Input: part model. Units: mm. Frame: model coordinates. Face numbers are marked on the shaded views. A direction names the side the tool comes from. Give positions to 0.01 mm unless a question says otherwise; leave off trailing zeros. Loops run counter-clockwise (first coordinate to the right, second up) from the corner with the lowest first, then second, coordinate; pieces in that order, holes last. Notation, with made-up numbers: M 9,42 L 51,42 A14 ccw 51,56 Z; hole C -39,6.25 d9. An arc over 180 degrees is marked long. One line per item, written item: value. Start each with the question number.
(1) Ray query, line 1 along X through (y, z) = (25, 0); line 2 along X through (y, z) = (33, -35); line 3 along Y through (x, z) = (0, 47.35). Return the intervals inside material, ascending. Write a range as from..to.
(2) Section A-A on y = 39.5. Output: boundary loops of the cut face in (x, z), plus the area to 3 significant figures.
(3) Section D-D on x = -17. Output: boundary loops of the cut face in (y, z), plus the area to 3 significant figures.
(4) Access query for the marked faces 1, 2 and 3. Directions: +Z, -Z, +X, -X, +Y, -Y. A direction counts if a zero-diameter tool reaches every point of the face in a straight line with its end or side. Return the directions, or none.
(5) Pull-direction query (X, two-part tool) for the marked faces 4, 5, 6 and 7; classes: released by +X, released by -X, zero draft, split by the parting line, or undercut.
(6) Section B-B on z = 0. Output: boundary loops of the cut face in (x, y).
(7) Pin query (flat end, axial travel): P1, Ø10.5, axis at x = -8.5, z = 21.5, coming from the +Y side; P2, Ø1, axis at y = 48.5, z = 14, coming from the +X side; P3, Ø22, axis at x = 3, y = 19.5, coming from the +Z side. Return the tip coordinate at first contact, or that it passes through.
(8) Section C-C on z = -41. Output: boundary loops of the cut face in (x, y), plus the area to 3 significant figures.
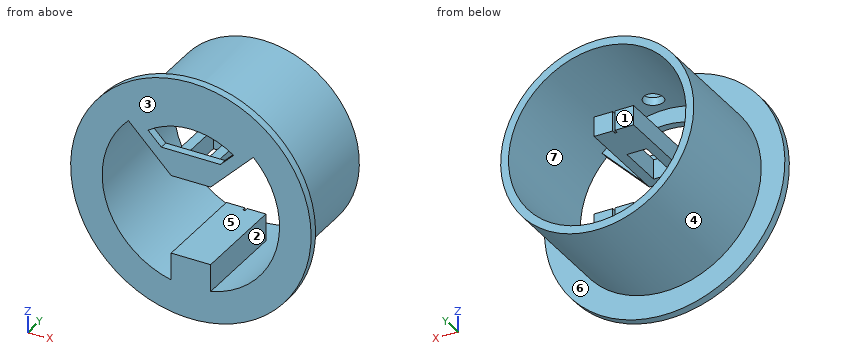
```python
from build123d import *

# Parameters (mm, degrees)
SKETCH1_R               = 61
SKETCH1_R_2             = 49
BOSS_EXTRUDE1_DEPTH     = 4
BOSS_EXTRUDE2_DEPTH     = 4
SKETCH1_5_R             = 49
SKETCH1_5_R_2           = 45
BOSS_EXTRUDE3_DEPTH     = 64.4
SKETCH1_8_W             = 20
SKETCH1_8_H             = 10
BOSS_EXTRUDE4_DEPTH     = 49.5
CUT_EXTRUDE1_REACH      = 115.669
SKETCH2_W               = 10
SKETCH2_H               = 24
CUT_EXTRUDE2_REACH      = 115.669
CUT_EXTRUDE2_END_RADIUS = 49
SKETCH3_R               = 5
CUT_EXTRUDE4_START      = -2
CUT_EXTRUDE4_DEPTH      = 2
SKETCH5_W               = 1.2
SKETCH5_H               = 10
CUT_EXTRUDE5_DEPTH      = 2


with BuildPart() as part:
    # Sketch1 → Boss-Extrude1 (new body)
    with BuildSketch(Plane(origin=(0, 0, 0), x_dir=(1, 0, 0), z_dir=(0, 1, 0))):
        with Locations(Location((0, 0, 0), (0, 0, 270))):
            Circle(SKETCH1_R)
        with Locations(Location((0, 0, 0), (0, 0, 270))):
            Circle(SKETCH1_R_2, mode=Mode.SUBTRACT)
    extrude(amount=BOSS_EXTRUDE1_DEPTH)



with BuildPart() as body_2:
    # Sketch1<4> → Boss-Extrude2 (new body)
    with BuildSketch(Plane(origin=(0, 0, 0), x_dir=(1, 0, 0), z_dir=(0, 1, 0))):
        with BuildLine():
            Line((31.692781496, -31.946323748), (10, -10.08))
            Line((10, -10.08), (10, -20.08))
            Line((10, -20.08), (-10, -20.08))
            Line((-10, -20.08), (-10, -10.08))
            Line((-10, -10.08), (-31.692781496, -31.946323748))
            ThreePointArc((-31.692781496, -31.946323748), (0, -45), (31.692781496, -31.946323748))
        make_face()
        with BuildLine():
            Line((-21.677506364, -29.984758092), (-15, -23.253831677))
            Line((-15, -23.253831677), (15, -23.253831677))
            Line((15, -23.253831677), (21.677506364, -29.984758092))
            ThreePointArc((21.677506364, -29.984758092), (0, -37), (-21.677506364, -29.984758092))
        make_face(mode=Mode.SUBTRACT)
    extrude(amount=BOSS_EXTRUDE2_DEPTH)


with BuildPart() as part_1:
    add(part.part)

    add(body_2.part)  # Boss-Extrude3 merges body 2
    # Sketch1<5> → Boss-Extrude3 (add)
    with BuildSketch(Plane(origin=(0, 0, 0), x_dir=(1, 0, 0), z_dir=(0, 1, 0))):
        with Locations(Location((0, 0, 0), (0, 0, 270))):
            Circle(SKETCH1_5_R)
        with Locations(Location((0, 0, 0), (0, 0, 314.77173117))):
            Circle(SKETCH1_5_R_2, mode=Mode.SUBTRACT)
    extrude(amount=BOSS_EXTRUDE3_DEPTH)

    # Sketch1<8> → Boss-Extrude4 (add)
    with BuildSketch(Plane(origin=(0, 0, 0), x_dir=(1, 0, 0), z_dir=(0, 1, 0))):
        with BuildLine():
            Line((-10, 30), (0, 30))
            Line((0, 30), (10, 30))
            Line((10, 30), (10, 43.874821937))
            ThreePointArc((10, 43.874821937), (0, 45), (-10, 43.874821937))
            Line((-10, 43.874821937), (-10, 30))
        make_face()
        with Locations((0, -15.08)):
            Rectangle(SKETCH1_8_W, SKETCH1_8_H)
    extrude(amount=BOSS_EXTRUDE4_DEPTH)

    # Sketch2 → Cut-Extrude1 (cut, up to next)
    with BuildSketch(Plane(origin=(0, 0, 10.08), x_dir=(-1, 0, 0), z_dir=(0, 0, -1)), mode=Mode.PRIVATE) as cut_extrude1_sk1:
        with Locations((0, 17)):
            Rectangle(SKETCH2_W, SKETCH2_H)
    cut_extrude1_tool1 = extrude(cut_extrude1_sk1.sketch, amount=-CUT_EXTRUDE1_REACH, mode=Mode.PRIVATE) & part_1.part
    add(cut_extrude1_tool1.solids().sort_by_distance((0, 17, 10.08))[0], mode=Mode.SUBTRACT)

    # Cut-Extrude2: up to this cylinder (the profile starts inside it)
    cut_extrude2_end = Plane(origin=(0, 14, 0), z_dir=(0, -1, 0)) * Cylinder(CUT_EXTRUDE2_END_RADIUS, 330.338, mode=Mode.PRIVATE)
    # Sketch3 → Cut-Extrude2 (cut, up to the surface)
    with BuildSketch(Plane(origin=(0, 0, 10.08), x_dir=(-1, 0, 0), z_dir=(0, 0, -1)), mode=Mode.PRIVATE) as cut_extrude2_sk1:
        with Locations((0, 14)):
            Circle(SKETCH3_R)
    cut_extrude2_tool1 = extrude(cut_extrude2_sk1.sketch, amount=-CUT_EXTRUDE2_REACH, mode=Mode.PRIVATE) & cut_extrude2_end
    add(cut_extrude2_tool1.solids().sort_by_distance((0, 14, 10.08))[0], mode=Mode.SUBTRACT)

    # Sketch4 → Cut-Extrude4 (cut)
    with BuildSketch(Plane(origin=(0, 49.5, 0), x_dir=(1, 0, 0), z_dir=(0, 1, 0)).offset(CUT_EXTRUDE4_START)):
        with BuildLine():
            Line((-0.6, 44.995999822), (-0.6, 30))
            Line((-0.6, 30), (0.6, 30))
            Line((0.6, 30), (0.6, 44.995999822))
            Line((0.6, 44.995999822), (0, 45))
            ThreePointArc((0, 45), (-0.300006667, 44.998999944), (-0.6, 44.995999822))
        make_face()
    extrude(amount=CUT_EXTRUDE4_DEPTH, mode=Mode.SUBTRACT)

    # Sketch5 → Cut-Extrude5 (cut)
    with BuildSketch(Plane(origin=(0, 49.5, 0), x_dir=(1, 0, 0), z_dir=(0, 1, 0))):
        with Locations((0, -15.08)):
            Rectangle(SKETCH5_W, SKETCH5_H)
    extrude(amount=-CUT_EXTRUDE5_DEPTH, mode=Mode.SUBTRACT)


solid = part_1.part
```
Output values:
1. line 1: x = -49..-45, 45..49
1. line 2: x = -34.29..-28.28, -10..10, 28.28..34.29
1. line 3: y = 0..9, 19..64.4
2. outline: C 0,0 d98; M -10,10.08 L 10,10.08 L 10,20.08 L -10,20.08 Z; hole M -10,-43.87 L -10,-30 L 10,-30 L 10,-43.87 A45 ccw long Z
2. area: 1,670 mm²
3. outline: M 0,-58.58 L 4,-58.58 L 4,-45.96 L 64.4,-45.96 L 64.4,-41.67 L 0,-41.67 Z; M 0,17.14 L 4,17.14 L 4,25.27 L 0,25.27 Z; M 0,32.86 L 4,32.86 L 4,41.67 L 64.4,41.67 L 64.4,45.96 L 4,45.96 L 4,58.58 L 0,58.58 Z
3. area: 721 mm²
4. face 1: +Y
4. face 2: +Y, -Y
4. face 3: +Z, -Z, +X, -X, -Y
5. face 4: split by the parting line
5. face 5: undercut
5. face 6: zero draft
5. face 7: undercut
6. outline: M -61,0 L -45,0 L -45,64.4 L -49,64.4 L -49,4 L -61,4 Z; M 45,0 L 61,0 L 61,4 L 49,4 L 49,64.4 L 45,64.4 Z
7. P1: stops at y = 49.5
7. P2: stops at x = 47.1
7. P3: stops at z = 49
8. outline: M -45.17,0 L -18.55,0 L -18.55,64.4 L -26.83,64.4 L -26.83,4 L -45.17,4 Z; M -10,0 L 10,0 L 10,49.5 L 0.6,49.5 L 0.6,47.5 L -0.6,47.5 L -0.6,49.5 L -10,49.5 Z; M 18.55,0 L 45.17,0 L 45.17,4 L 26.83,4 L 26.83,64.4 L 18.55,64.4 Z
8. area: 2,200 mm²
